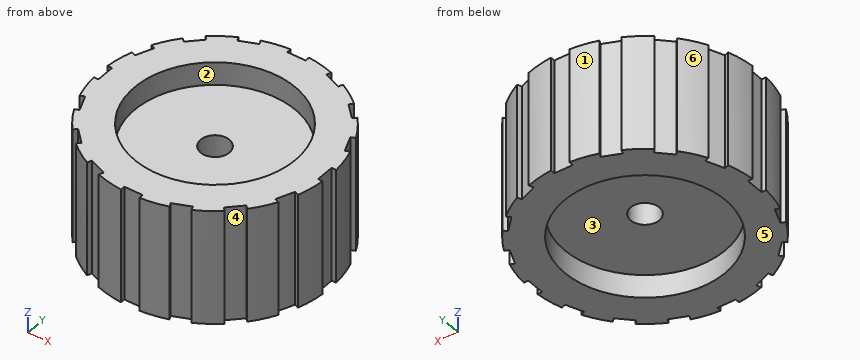
```python
from build123d import *

# Parameters (mm, degrees)
SKETCH1_R           = 17.78
BOSS_EXTRUDE2_DEPTH = 25.4
SKETCH1_3_R         = 17.78
SKETCH1_3_R_2       = 3.175
BOSS_EXTRUDE3_DEPTH = 20.32
SKETCH1_4_R         = 17.78
SKETCH1_4_R_2       = 3.175
CUT_EXTRUDE1_DEPTH  = 5.08


with BuildPart() as part:
    # Sketch1 → Boss-Extrude2 (new body)
    with BuildSketch(Plane.XY):
        with BuildLine():
            Line((11.566327956, 22.613713928), (11.177521588, 21.675052323))
            Line((11.177521588, 21.675052323), (7.422875168, 23.230277792))
            Line((7.422875168, 23.230277792), (7.811681536, 24.168939397))
            ThreePointArc((7.811681536, 24.168939397), (4.955294179, 24.911946122), (2.032, 25.318589534))
            Line((2.032, 25.318589534), (2.032, 24.302589534))
            Line((2.032, 24.302589534), (-2.032, 24.302589534))
            Line((-2.032, 24.302589534), (-2.032, 25.318589534))
            ThreePointArc((-2.032, 25.318589534), (-4.955294179, 24.911946122), (-7.811681536, 24.168939397))
            Line((-7.811681536, 24.168939397), (-7.422875168, 23.230277792))
            Line((-7.422875168, 23.230277792), (-11.177521588, 21.675052323))
            Line((-11.177521588, 21.675052323), (-11.566327956, 22.613713928))
            ThreePointArc((-11.566327956, 22.613713928), (-14.111483919, 21.119328152), (-16.46610537, 19.339787329))
            Line((-16.46610537, 19.339787329), (-15.747684881, 18.621366839))
            Line((-15.747684881, 18.621366839), (-18.621366839, 15.747684881))
            Line((-18.621366839, 15.747684881), (-19.339787329, 16.46610537))
            ThreePointArc((-19.339787329, 16.46610537), (-21.119328152, 14.111483919), (-22.613713928, 11.566327956))
            Line((-22.613713928, 11.566327956), (-21.675052323, 11.177521588))
            Line((-21.675052323, 11.177521588), (-23.230277792, 7.422875168))
            Line((-23.230277792, 7.422875168), (-24.168939397, 7.811681536))
            ThreePointArc((-24.168939397, 7.811681536), (-24.911946122, 4.955294179), (-25.318589534, 2.032))
            Line((-25.318589534, 2.032), (-24.302589534, 2.032))
            Line((-24.302589534, 2.032), (-24.302589534, -2.032))
            Line((-24.302589534, -2.032), (-25.318589534, -2.032))
            ThreePointArc((-25.318589534, -2.032), (-24.911946122, -4.955294179), (-24.168939397, -7.811681536))
            Line((-24.168939397, -7.811681536), (-23.230277792, -7.422875168))
            Line((-23.230277792, -7.422875168), (-21.675052323, -11.177521588))
            Line((-21.675052323, -11.177521588), (-22.613713928, -11.566327956))
            ThreePointArc((-22.613713928, -11.566327956), (-21.119328152, -14.111483919), (-19.339787329, -16.46610537))
            Line((-19.339787329, -16.46610537), (-18.621366839, -15.747684881))
            Line((-18.621366839, -15.747684881), (-15.747684881, -18.621366839))
            Line((-15.747684881, -18.621366839), (-16.46610537, -19.339787329))
            ThreePointArc((-16.46610537, -19.339787329), (-14.111483919, -21.119328152), (-11.566327956, -22.613713928))
            Line((-11.566327956, -22.613713928), (-11.177521588, -21.675052323))
            Line((-11.177521588, -21.675052323), (-7.422875168, -23.230277792))
            Line((-7.422875168, -23.230277792), (-7.811681536, -24.168939397))
            ThreePointArc((-7.811681536, -24.168939397), (-4.955294179, -24.911946122), (-2.032, -25.318589534))
            Line((-2.032, -25.318589534), (-2.032, -24.302589534))
            Line((-2.032, -24.302589534), (2.032, -24.302589534))
            Line((2.032, -24.302589534), (2.032, -25.318589534))
            ThreePointArc((2.032, -25.318589534), (4.955294179, -24.911946122), (7.811681536, -24.168939397))
            Line((7.811681536, -24.168939397), (7.422875168, -23.230277792))
            Line((7.422875168, -23.230277792), (11.177521588, -21.675052323))
            Line((11.177521588, -21.675052323), (11.566327956, -22.613713928))
            ThreePointArc((11.566327956, -22.613713928), (14.111483919, -21.119328152), (16.46610537, -19.339787329))
            Line((16.46610537, -19.339787329), (15.747684881, -18.621366839))
            Line((15.747684881, -18.621366839), (18.621366839, -15.747684881))
            Line((18.621366839, -15.747684881), (19.339787329, -16.46610537))
            ThreePointArc((19.339787329, -16.46610537), (21.119328152, -14.111483919), (22.613713928, -11.566327956))
            Line((22.613713928, -11.566327956), (21.675052323, -11.177521588))
            Line((21.675052323, -11.177521588), (23.230277792, -7.422875168))
            Line((23.230277792, -7.422875168), (24.168939397, -7.811681536))
            ThreePointArc((24.168939397, -7.811681536), (24.911946122, -4.955294179), (25.318589534, -2.032))
            Line((25.318589534, -2.032), (24.302589534, -2.032))
            Line((24.302589534, -2.032), (24.302589534, 2.032))
            Line((24.302589534, 2.032), (25.318589534, 2.032))
            ThreePointArc((25.318589534, 2.032), (24.911946122, 4.955294179), (24.168939397, 7.811681536))
            Line((24.168939397, 7.811681536), (23.230277792, 7.422875168))
            Line((23.230277792, 7.422875168), (21.675052323, 11.177521588))
            Line((21.675052323, 11.177521588), (22.613713928, 11.566327956))
            ThreePointArc((22.613713928, 11.566327956), (21.119328152, 14.111483919), (19.339787329, 16.46610537))
            Line((19.339787329, 16.46610537), (18.621366839, 15.747684881))
            Line((18.621366839, 15.747684881), (15.747684881, 18.621366839))
            Line((15.747684881, 18.621366839), (16.46610537, 19.339787329))
            ThreePointArc((16.46610537, 19.339787329), (14.111483919, 21.119328152), (11.566327956, 22.613713928))
        make_face()
        Circle(SKETCH1_R, mode=Mode.SUBTRACT)
    extrude(amount=BOSS_EXTRUDE2_DEPTH)

    # Sketch1<3> → Boss-Extrude3 (add)
    with BuildSketch(Plane.XY):
        Circle(SKETCH1_3_R)
        Circle(SKETCH1_3_R_2, mode=Mode.SUBTRACT)
    extrude(amount=BOSS_EXTRUDE3_DEPTH)

    # Sketch1<4> → Cut-Extrude1 (cut)
    with BuildSketch(Plane.XY):
        Circle(SKETCH1_4_R)
        Circle(SKETCH1_4_R_2, mode=Mode.SUBTRACT)
    extrude(amount=CUT_EXTRUDE1_DEPTH, mode=Mode.SUBTRACT)


solid = part.part
```
Read the model definition and answer for the solid it produces. Units are mm, in the model's axes. Face numbers are marked on the shaded views. A direction names the side the tool comes from. Coordinates: 2 decimals unless noted, no trailing zeros. Write each loop counter-clockwise with the first axis right and the second up, starting at its lowest first coordinate (ties: lowest second). Pieces come first, ordered by that corner, then holes. Notation, with made-up numbers: (47.5, 13) - (54.5, 13) arc R32 cw to (54.5, 51) - close; hole circle Ø5 at (60.25, 56.25). An arc over 180 degrees is marked (long way). Answer as a JSON object with one key per item and string values. Group by question number.
1. A cutting plane is placed at A-A (y = 0). Determine the outline of the cut face in (x, z) (3 decimals).
2. A cutting plane is placed at D-D (y = -9). Determine the outline of the cut face in (x, z).
3. Consider L1, parallel to Y at x = 0, z = 3.35; L2, parallel to Y at x = 0, z = 15 (3 decimals); L3, parallel to Z at x = -7, y = -12. Determine where each line is inside the solid, lowest interval first. Write a range as [from, to].
4. Each of these flat-tipped pins is pushed along its axis until it touches: P1, Ø1.1, axis at x = 24.5, z = 15.5, coming from the +Y side; P2, Ø5, axis at y = 8.5, z = 21.5, coming from the +X side; P3, Ø18, axis at x = -1, y = -8, coming from the +Z side. Where does it stop, or does it pass through?
5. Which of the six approach directions +Z, -Z, +X, -X, +Y, -Y give full straight-line access (tool end or side, diameter ignored) to the marked faces 1, 2 and 3?
6. A cutting plane is placed at C-C (x = 10.5). Determine the outline of the cut face in (y, z), plus the area to 3 significant figures.
7. The mould has two halves that part along Y. Classify the marked faces 4, 5 and 6: +Y half, -Y half, draft (parallel to the pull), parting line (faces both ways), or undercut.
Worked out:
{
 "1": {"outline": "(-24.303, 0) - (-17.78, 0) - (-17.78, 5.08) - (-3.175, 5.08) - (-3.175, 20.32) - (-17.78, 20.32) - (-17.78, 25.4) - (-24.303, 25.4) - close; (3.175, 5.08) - (17.78, 5.08) - (17.78, 0) - (24.303, 0) - (24.303, 25.4) - (17.78, 25.4) - (17.78, 20.32) - (3.175, 20.32) - close"},
 "2": {"outline": "(-22.58, 0) - (-15.33, 0) - (-15.33, 5.08) - (15.33, 5.08) - (15.33, 0) - (22.58, 0) - (22.58, 25.4) - (15.33, 25.4) - (15.33, 20.32) - (-15.33, 20.32) - (-15.33, 25.4) - (-22.58, 25.4) - close"},
 "3": {"L1": "y = [-24.3, -17.78], [17.78, 24.3]", "L2": "y = [-24.303, -3.175], [3.175, 24.303]", "L3": "z = [5.08, 20.32]"},
 "4": {"P1": "stops at y = 7.81", "P2": "stops at x = 24.68", "P3": "stops at z = 20.32"},
 "5": {"face 1": "+Z, -Z, -X, +Y", "face 2": "+Z", "face 3": "-Z"},
 "6": {"outline": "(-21.96, 0) - (-14.35, 0) - (-14.35, 5.08) - (14.35, 5.08) - (14.35, 0) - (21.96, 0) - (21.96, 25.4) - (14.35, 25.4) - (14.35, 20.32) - (-14.35, 20.32) - (-14.35, 25.4) - (-21.96, 25.4) - close", "area": "824 mm²"},
 "7": {"face 4": "undercut", "face 5": "draft", "face 6": "+Y half"}
}
